Autodesk Inventor part; units mm, degrees
ref_plane "Start Plane" through (0, 0, 0) normal (0, 0, 1) x (1, 0, 0)
ref_plane "End Plane" through (0, 0, 50.8) normal (0, 0, 1) x (1, 0, 0)
ref_plane "YZ Plane" through (0, 0, 0) normal (1, 0, 0) x (0, 1, 0)
ref_plane "Start Plane" through (0, 0, 0) normal (0, 0, 1) x (1, 0, 0)
ref_plane "End Plane" through (0, 0, 50.8) normal (0, 0, 1) x (1, 0, 0)
sketch "Sketch1" plane through (0, 0, 0) normal (0, 0, 1) x (1, 0, 0)
  line L0 (-12.7, 12.7) -> (12.7, 12.7)
  line L1 (12.7, 12.7) -> (12.7, -12.7)
  line L2 (12.7, -12.7) -> (-12.7, -12.7)
  line L3 (-12.7, -12.7) -> (-12.7, 12.7)
  line L4 (9.525, 9.525) -> (-9.525, 9.525)
  line L5 (-9.525, 9.525) -> (-9.525, -9.525)
  line L6 (-9.525, -9.525) -> (9.525, -9.525)
  line L7 (9.525, -9.525) -> (9.525, 9.525)
  point P0 (0, 0)
  point P1 (0, 12.7)
  point P2 (-12.7, 0)
  dimension "width" = 25.4
  dimension "d1" = 3.175
extrude "Body" add sketch "Sketch1" along normal up to surface (50.8 mm away) from surface at 0
sketch "Sketch4" plane through (0, 0, 0) normal (0, 0, 1) x (1, 0, 0)
  line L0 (0, 0) -> (10, 0)
ref_plane "Work Plane4" through (0, 0, 0) normal (0, -1, 0) x (1, 0, 0)
sketch "Sketch5" plane through (0, 0, 0) normal (0, -1, 0) x (1, 0, 0)
  line L0 (-17.78, 0) -> (17.78, 0)
  line L1 (-17.78, 50.8) -> (17.78, 50.8)
  dimension "d9" = 50.8
equation "\"G_OFFSET_START\" = 0"
equation "\"G_OFFSET_END\" = 0"
equation "\"d5\" = length + G_OFFSET_END"
equation "\"G_L\" = d9"
properties part number "Square Tube Profile"
Read the model definition and answer for the solid it produces. Units are mm, in the model's axes. A direction names the side the tool comes from. Round coordinates to 2 decimals unless told otherwise and drop trailing zeros. Write each loop counter-clockwise with the first axis right and the second up, starting at its lowest first coordinate (ties: lowest second). Pieces come first, ordered by that corner, then holes.
Q1. Find section C-C on z = 15. Determine the outline of the cut face in (x, y) (3 decimals).
Values:
outline: (-12.7, -12.7) - (12.7, -12.7) - (12.7, 12.7) - (-12.7, 12.7) - close; hole (-9.525, -9.525) - (9.525, -9.525) - (9.525, 9.525) - (-9.525, 9.525) - close
Q2. The mould has two halves that part along Y. Classify faces 3 (the face through (11, 0, 50.8)), 4 (the face through (-9.525, 0, 25)), 5 (the face through (0, -12.7, 25)): released by +Y, released by -Y, zero draft, split by the parting line, or undercut.
Values:
face 3: zero draft
face 4: undercut
face 5: released by -Y
Q3. Find section A-A on x = -7. Determine the outline of the cut face in (y, z) (3 decimals), and give its area (3 significant figures).
Values:
outline: (-12.7, 0) - (-9.525, 0) - (-9.525, 50.8) - (-12.7, 50.8) - close; (9.525, 0) - (12.7, 0) - (12.7, 50.8) - (9.525, 50.8) - close
area: 323 mm2
Q4. A tool of negligible diameter and unlimited length cuts with its end or side. For faces 1 (the face through (0, 9.525, 25)), 2 (the face through (12.7, 0, 25)), from which of +Z, -Z, +X, -X, +Y, -Y can it reach the whole face along a straight path? Write none if from no direction.
Values:
face 1: +Z, -Z
face 2: +Z, -Z, +X, +Y, -Y
Q5. A straight line is drawn through the part: line 1 (Y direction, x = -7.75, z = 43) (3 decimals). Find the intervals that lie inside material, in ascending order.
Values:
line 1: y = -12.7 to -9.525, 9.525 to 12.7
